Build history of the part. All positions in model axes, mm. Face numbers are marked on the shaded views. A direction names the side the tool comes from. Round coordinates to 2 decimals unless told otherwise and drop trailing zeros. Order: outer loops, then holes, each group sorted by start corner. A loop starts at its lowest first (then second) coordinate and runs counter-clockwise, first axis right, second up. Notation, with made-up numbers: (87.5, 70) -> (140.5, 70) arc R25 cw to (140.5, 89) -> close; hole circle Ø7 at (71.25, 58.5). An arc over 180 degrees is marked (long way). Use a Markdown table: item, result. Add a question column.
Item 1: Slice it at D-D, the plane y = 11.75. Give the cut face in (x, z).
Item 2: 3-axis set-ups, long thin cutter, end or side, ignore diameter. For the marked faces 1 and 2: which of +Z, -Z, +X, -X, +Y, -Y reach the whole face in a straight line?
Item 3: Slice it at B-B, the plane y = 5.5. Give the cut face in (x, z), plus the area to 3 significant figures.
Item 4: Probe L1, parallel to Z at x = 7.5, y = 5.3; L2, parallel to Y at x = 7.5, z = 7.15; L3, parallel to Y at x = 7.75, z = 10. List the from-to ranges inside material, lowest first.
Item 5: Slice it at A-A, the plane x = 9.5. Give the cut face in (y, z), plus the area to 3 significant figures.
Item 6: Slice it at C-C, the plane z = 11. Give the cut face in (x, y), plus the area to 3 significant figures.
Item 7: Two-plate mould, pull along X, no slides. Class the marked faces 3, 4, 5 and 6: released by +X, released by -X, zero draft, split by the parting line, or undercut.
Item 8: Pin check, flat tips, straight feed: pin 1 (0.7 mm diameter, centred on y = 7.5, z = 10.5, fed in from +X); pin 2 (1.7 mm diameter, centred on x = 9.5, z = 5, fed in from -Y); pin 3 (3 mm diameter, centred on x = 7.5, z = 4.57, fed in from +Y). Stop position of each tip, or through.
from build123d import *

# Parameters (mm, degrees)
F0_W     = 15
F0_H     = 15
F1_DEPTH = 15
F2_W     = 5.503
F2_H     = 2.3
F2_W_2   = 2.3
F2_H_2   = 5.503
F3_DEPTH = 11.5
F5_D     = 3.4
F5_DEPTH = 12
F5_TIP   = 1.0214630523
F7_D     = 3.4
F7_DEPTH = 12
F7_TIP   = 1.0214630523


with BuildPart() as f1:
    # F0 (on Top) → F1 (new body)
    with BuildSketch(Plane.XY):
        with Locations((7.5, 7.5)):
            Rectangle(F0_W, F0_H)
    extrude(amount=F1_DEPTH)

    # F2 (on face) → F3 (cut)
    with BuildSketch(Plane.YZ.offset(15)):
        with Locations((7.5, 10.4661304504)):
            Rectangle(F2_W, F2_H)
        with Locations((10.8725838363, 4.5725819655)):
            Rectangle(F2_W_2, F2_H_2)
    extrude(amount=-F3_DEPTH, mode=Mode.SUBTRACT)

    # F5
    with Locations(Plane.XY.offset(15)):
        with Locations((7.5, 7.5)):
            Hole(F5_D / 2, depth=F5_DEPTH)
            with Locations((0, 0, -(F5_DEPTH + F5_TIP / 2))):  # 118° drill point
                Cone(0, F5_D / 2, F5_TIP, mode=Mode.SUBTRACT)

    # F7
    with Locations(Plane(origin=(0, 15, 0), x_dir=(-1, 0, 0), z_dir=(0, 1, 0))):
        with Locations((-7.5, 4.5725819655)):
            Hole(F7_D / 2, depth=F7_DEPTH)
            with Locations((0, 0, -(F7_DEPTH + F7_TIP / 2))):  # 118° drill point
                Cone(0, F7_D / 2, F7_TIP, mode=Mode.SUBTRACT)


solid = f1.part
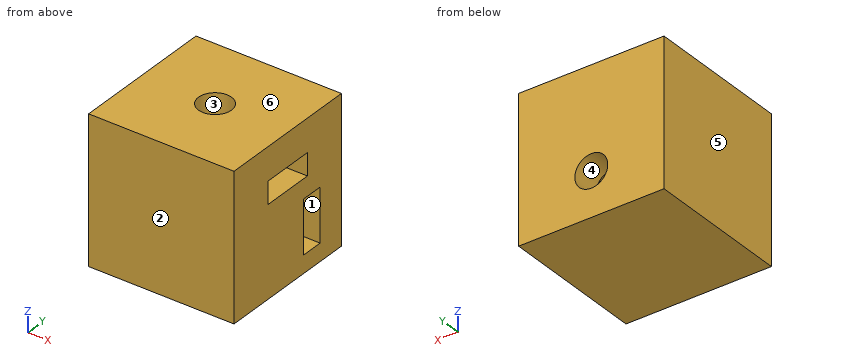
Check sheet entries:
| question | item | result |
|---|---|---|
| 1 | outline | (0, 0) -> (15, 0) -> (15, 1.82) -> (3.5, 1.82) -> (3.5, 7.32) -> (15, 7.32) -> (15, 15) -> (0, 15) -> close |
| 2 | face 1 | +X |
| 2 | face 2 | +Z, -Z, +X, -X, -Y |
| 3 | outline | (0, 0) -> (15, 0) -> (15, 9.32) -> (3.5, 9.32) -> (3.5, 11.62) -> (15, 11.62) -> (15, 15) -> (0, 15) -> close; hole circle Ø3.4 at (7.5, 4.57) |
| 3 | area | 189 mm2 |
| 4 | L1 | 0 to 2.87, 6.27 to 9.32, 11.62 to 15 |
| 4 | L2 | 0 to 5.8, 9.2 to 9.72, 12.02 to 15 |
| 4 | L3 | 0 to 4.75, 10.25 to 15 |
| 5 | outline | (0, 0) -> (15, 0) -> (15, 15) -> (0, 15) -> close; hole (4.75, 9.32) -> (10.25, 9.32) -> (10.25, 11.62) -> (4.75, 11.62) -> close; hole (9.72, 1.82) -> (12.02, 1.82) -> (12.02, 7.32) -> (9.72, 7.32) -> close |
| 5 | area | 200 mm2 |
| 6 | outline | (0, 0) -> (15, 0) -> (15, 4.75) -> (3.5, 4.75) -> (3.5, 10.25) -> (15, 10.25) -> (15, 15) -> (0, 15) -> close |
| 6 | area | 162 mm2 |
| 7 | face 3 | undercut |
| 7 | face 4 | undercut |
| 7 | face 5 | released by -X |
| 7 | face 6 | zero draft |
| 8 | pin 1 | x = 3.5 |
| 8 | pin 2 | y = 0 |
| 8 | pin 3 | y = 2.88 |
